The model under review builds one solid part; all positions refer to its coordinate system, in mm. Round coordinates to 2 decimals unless told otherwise and drop trailing zeros. Order: outer loops, then holes, each group sorted by start corner. A loop starts at its lowest first (then second) coordinate and runs counter-clockwise, first axis right, second up.
```python
from build123d import *

# Parameters (mm, degrees)
SKETCH2_R                        = 139.7
SKETCH2_R_2                      = 50.8
BOSS_EXTRUDE1_DEPTH              = 9.525
SKETCH3_R                        = 12.6746
SKETCH3_R_2                      = 6.35
CUT_EXTRUDE2_DEPTH               = 10.525
F_1_4_20_TAPPED_HOLE1_AT_2_COUNT = 2
F_1_4_20_TAPPED_HOLE1_AT_2_PITCH = 60.61075
F_1_4_20_TAPPED_HOLE1_AT_3_COUNT = 2
F_1_4_20_TAPPED_HOLE1_AT_3_PITCH = 104.980898485
F_1_4_20_TAPPED_HOLE1_AT_4_COUNT = 2
F_1_4_20_TAPPED_HOLE1_AT_4_PITCH = 121.2215
F_1_4_20_TAPPED_HOLE1_AT_5_COUNT = 2
F_1_4_20_TAPPED_HOLE1_AT_5_PITCH = 104.980898485
F_1_4_20_TAPPED_HOLE1_AT_6_COUNT = 2
F_1_4_20_TAPPED_HOLE1_AT_6_PITCH = 60.61075


with BuildPart() as part:
    # Sketch2 → Boss-Extrude1 (new body)
    with BuildSketch(Plane(origin=(0, 0, 0), x_dir=(1, 0, 0), z_dir=(0, 1, 0))):
        Circle(SKETCH2_R)
        Circle(SKETCH2_R_2, mode=Mode.SUBTRACT)
    extrude(amount=BOSS_EXTRUDE1_DEPTH)

    # Sketch3 → Cut-Extrude2 (cut, through all)
    with BuildSketch(Plane(origin=(0, 9.525, 0), x_dir=(1, 0, 0), z_dir=(0, 1, 0))):
        with Locations((0, 120.65)):
            Circle(SKETCH3_R)
        with Locations((120.65, 0)):
            Circle(SKETCH3_R)
        with Locations((0, -120.65)):
            Circle(SKETCH3_R)
        with Locations((-120.65, 0)):
            Circle(SKETCH3_R)
        with Locations((85.31243315, 85.31243315)):
            Circle(SKETCH3_R_2)
        with Locations((85.31243315, -85.31243315)):
            Circle(SKETCH3_R_2)
        with Locations((-85.31243315, -85.31243315)):
            Circle(SKETCH3_R_2)
        with Locations((-85.31243315, 85.31243315)):
            Circle(SKETCH3_R_2)
    extrude(amount=-CUT_EXTRUDE2_DEPTH, mode=Mode.SUBTRACT)

    # Sketch6 → 1/4-20 Tapped Hole1 (revolve, cut)
    with BuildSketch(Plane(origin=(-58.545488776, 9.525, -15.687216438), x_dir=(0, 0, 1), z_dir=(1, 0, 0))):
        Polygon((0, 0), (0, 9.525), (3.81, 9.525), (2.5527, 8.2677), (2.5527, 1.2573), (3.81, 0), align=None)
    f_1_4_20_tapped_hole1 = revolve(axis=Axis((-58.545488776, 15.875, -15.687216438), (0, -1, 0)), mode=Mode.SUBTRACT)

    # 1/4-20 Tapped Hole1 at 2: 1/4-20 Tapped Hole1 ×2
    with Locations(*[Vector(0.707106781, 0, -0.707106781) * (i * F_1_4_20_TAPPED_HOLE1_AT_2_PITCH) for i in range(1, F_1_4_20_TAPPED_HOLE1_AT_2_COUNT)]):
        add(f_1_4_20_tapped_hole1, mode=Mode.SUBTRACT)

    # 1/4-20 Tapped Hole1 at 3: 1/4-20 Tapped Hole1 ×2
    with Locations(*[Vector(0.965925826, 0, -0.258819045) * (i * F_1_4_20_TAPPED_HOLE1_AT_3_PITCH) for i in range(1, F_1_4_20_TAPPED_HOLE1_AT_3_COUNT)]):
        add(f_1_4_20_tapped_hole1, mode=Mode.SUBTRACT)

    # 1/4-20 Tapped Hole1 at 4: 1/4-20 Tapped Hole1 ×2
    with Locations(*[Vector(0.965925826, 0, 0.258819045) * (i * F_1_4_20_TAPPED_HOLE1_AT_4_PITCH) for i in range(1, F_1_4_20_TAPPED_HOLE1_AT_4_COUNT)]):
        add(f_1_4_20_tapped_hole1, mode=Mode.SUBTRACT)

    # 1/4-20 Tapped Hole1 at 5: 1/4-20 Tapped Hole1 ×2
    with Locations(*[Vector(0.707106781, 0, 0.707106781) * (i * F_1_4_20_TAPPED_HOLE1_AT_5_PITCH) for i in range(1, F_1_4_20_TAPPED_HOLE1_AT_5_COUNT)]):
        add(f_1_4_20_tapped_hole1, mode=Mode.SUBTRACT)

    # 1/4-20 Tapped Hole1 at 6: 1/4-20 Tapped Hole1 ×2
    with Locations(*[Vector(0.258819045, 0, 0.965925826) * (i * F_1_4_20_TAPPED_HOLE1_AT_6_PITCH) for i in range(1, F_1_4_20_TAPPED_HOLE1_AT_6_COUNT)]):
        add(f_1_4_20_tapped_hole1, mode=Mode.SUBTRACT)


solid = part.part
```
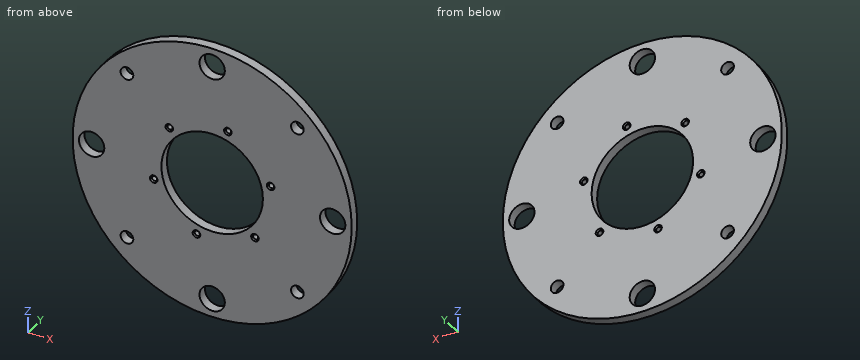
(1) Consider section C-C (x = -120.65). Write out the cut boundary in (y, z) (3 decimals), and give its area (3 significant figures).
Data:
outline: (0, -70.425) - (9.525, -70.425) - (9.525, -12.675) - (0, -12.675) - close; (0, 12.675) - (9.525, 12.675) - (9.525, 70.425) - (0, 70.425) - close
area: 1,100 mm2
(2) To check wall thickness, follow probe 1 along Z at (x, y) = (0, 3.25); probe 2 along X at (y, z) = (8, 80.5). State the ranges of each line that lie inside material, in increasing order.
Data:
probe 1: z = -139.7 to -133.32, -107.98 to -50.8, 50.8 to 107.98, 133.32 to 139.7
probe 2: x = -114.17 to -89.46, -81.17 to 81.17, 89.46 to 114.17
(3) Consider section B-B (z = 0). Write out the cut boundary in (x, y) (3 decimals).
Data:
outline: (-139.7, 0) - (-133.325, 0) - (-133.325, 9.525) - (-139.7, 9.525) - close; (-107.975, 0) - (-50.8, 0) - (-50.8, 9.525) - (-107.975, 9.525) - close; (50.8, 0) - (107.975, 0) - (107.975, 9.525) - (50.8, 9.525) - close; (133.325, 0) - (139.7, 0) - (139.7, 9.525) - (133.325, 9.525) - close
(4) Insertion check: pin 1 (20.5 mm diameter, centred on x = 0, z = -120.65, fed in from +Y); pin 2 (5 mm diameter, centred on y = 8.5, z = 28, fed in from +X); pin 3 (6 mm diameter, centred on x = -58.55, z = -15.69, fed in from -Y); pin 4 (6.5 mm diameter, centred on x = -15.69, z = -58.55, fed in from -Y). Each pin has a flat end and moves straight along its axis. Give the tip position at first contact, or say it passes through.
Data:
pin 1: passes through
pin 2: stops at x = 137.35
pin 3: stops at y = 0.8
pin 4: stops at y = 0.55
(5) Consider section A-A (x = 0). Write out the cut boundary in (y, z) (3 decimals), and give its area (3 significant figures).
Data:
outline: (0, -139.7) - (9.525, -139.7) - (9.525, -133.325) - (0, -133.325) - close; (0, -107.975) - (9.525, -107.975) - (9.525, -50.8) - (0, -50.8) - close; (0, 50.8) - (9.525, 50.8) - (9.525, 107.975) - (0, 107.975) - close; (0, 133.325) - (9.525, 133.325) - (9.525, 139.7) - (0, 139.7) - close
area: 1,210 mm2
(6) Consider section D-D (y = 5). State how many separate pieces and enclosed holes the cut face has, and give its area (3 significant figures).
Data:
separate pieces: 1
enclosed holes: 15
area: 50,600 mm2
